Build history of the part. All positions in model axes, mm. Face numbers are marked on the shaded views. A direction names the side the tool comes from. Round coordinates to 2 decimals unless told otherwise and drop trailing zeros. Write each loop counter-clockwise with the first axis right and the second up, starting at its lowest first coordinate (ties: lowest second). Pieces come first, ordered by that corner, then holes. Notation, with made-up numbers: (-31, 54.5) -> (-17, 54.5) arc R26 ccw to (-17, 84.5) -> close; hole circle Ø1 at (26.25, -33). An arc over 180 degrees is marked (long way). Answer in a Markdown table with one row per item. Add a question column.
from build123d import *

# Parameters (mm, degrees)
SKETCH1_R           = 3
SKETCH1_R_2         = 1.6
BOSS_EXTRUDE1_DEPTH = 3


with BuildPart() as part:
    # Sketch1 → Boss-Extrude1 (new body)
    with BuildSketch(Plane(origin=(0, 0, 0), x_dir=(1, 0, 0), z_dir=(0, 1, 0))):
        with BuildLine():
            Line((-4.898979486, 26), (-9.797958971, 2))
            ThreePointArc((-9.797958971, 2), (0, -10), (9.797958971, 2))
            Line((9.797958971, 2), (4.898979486, 26))
            ThreePointArc((4.898979486, 26), (0, 30), (-4.898979486, 26))
        make_face()
        with Locations(Location((0, 0, 0), (0, 0, 270))):
            Circle(SKETCH1_R, mode=Mode.SUBTRACT)
        with Locations(Location((0, 7, 0), (0, 0, 270))):
            Circle(SKETCH1_R_2, mode=Mode.SUBTRACT)
        with Locations(Location((7, 0, 0), (0, 0, 270))):
            Circle(SKETCH1_R_2, mode=Mode.SUBTRACT)
        with Locations(Location((0, -7, 0), (0, 0, 270))):
            Circle(SKETCH1_R_2, mode=Mode.SUBTRACT)
        with Locations(Location((-7, 0, 0), (0, 0, 270))):
            Circle(SKETCH1_R_2, mode=Mode.SUBTRACT)
        with BuildLine():
            Line((1.6, 25), (1.6, 20))
            ThreePointArc((1.6, 20), (0, 18.4), (-1.6, 20))
            Line((-1.6, 20), (-1.6, 25))
            ThreePointArc((-1.6, 25), (0, 26.6), (1.6, 25))
        make_face(mode=Mode.SUBTRACT)
    extrude(amount=BOSS_EXTRUDE1_DEPTH)


solid = part.part
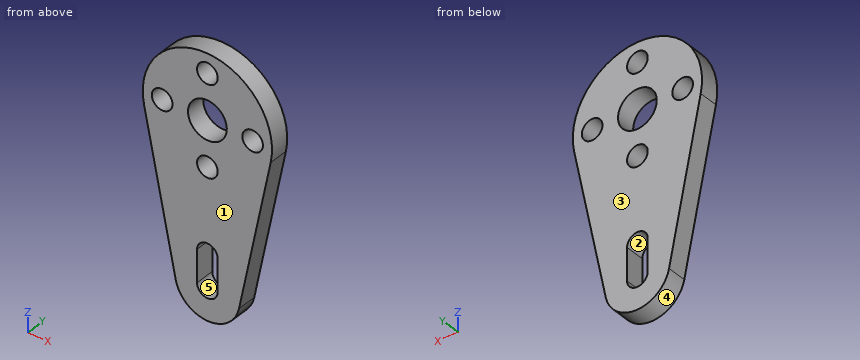
(1) Drop flat-ended pins along their axis: P1, Ø1, axis at y = 1.5, z = -25.5, coming from the +X side; P2, Ø1.5, axis at x = 5.5, y = 2, coming from the +Z side; P3, Ø1.5, axis at y = 1, z = -22, coming from the +X side. Give the stop position or say it passes through.
(2) Saw through at C-C (z = -6). List the corners of the cut face in (x, y).
(3) Probe line 1 along X through (y, z) = (1.7, 0); line 2 along Z through (x, y) = (0.25, 1.7); line 3 along Z through (x, y) = (1.75, 1.35). List the from-to ranges inside material, lowest first.
(4) Saw through at A-A (y = 1.15). List the corners of the cut face in (x, z).
(5) Saw through at B-B (x = 0). List the corners of the cut face in (y, z), plus the area to 3 significant figures.
(6) Saw through at D-D (x = -7). List the corners of the cut face in (y, z).
(7) Which spindle directions (+Z, -Z, +X, -X, +Y, -Y) get a long thin tool onto all of the face, cutting with end or side? Do the marked faces 1 and 2. Say none if no direction does.
(8) Mould opens along Z. For the marked faces 3, 4 and 5 say: pulls with the +Z half, pulls with the -Z half, needs draft (parallel to the pull), parting line crosses it, or undercut.
Answer sheet:
| question | item | result |
|---|---|---|
| 1 | P1 | stops at x = 5.1 |
| 1 | P2 | stops at z = 8.8 |
| 1 | P3 | stops at x = 5.87 |
| 2 | outline | (-8.98, 0) -> (-1.25, 0) -> (-1.25, 3) -> (-8.98, 3) -> close; (1.25, 0) -> (8.98, 0) -> (8.98, 3) -> (1.25, 3) -> close |
| 3 | line 1 | x = -10 to -8.6, -5.4 to -3, 3 to 5.4, 8.6 to 10 |
| 3 | line 2 | z = -29.99 to -26.58, -18.42 to -8.58, -5.42 to -2.99, 2.99 to 5.42, 8.58 to 10 |
| 3 | line 3 | z = -29.68 to -2.44, 2.44 to 9.85 |
| 4 | outline | (-9.8, -2) -> (-4.9, -26) arc R5 ccw to (4.9, -26) -> (9.8, -2) arc R10 ccw (long way) to start; hole circle Ø3.2 at (-7, 0); hole circle Ø6 at (0, 0); hole (-1.6, -25) arc R1.6 ccw to (1.6, -25) -> (1.6, -20) arc R1.6 ccw to (-1.6, -20) -> close; hole circle Ø3.2 at (0, -7); hole circle Ø3.2 at (0, 7); hole circle Ø3.2 at (7, 0) |
| 5 | outline | (0, -30) -> (3, -30) -> (3, -26.6) -> (0, -26.6) -> close; (0, -18.4) -> (3, -18.4) -> (3, -8.6) -> (0, -8.6) -> close; (0, -5.4) -> (3, -5.4) -> (3, -3) -> (0, -3) -> close; (0, 3) -> (3, 3) -> (3, 5.4) -> (0, 5.4) -> close; (0, 8.6) -> (3, 8.6) -> (3, 10) -> (0, 10) -> close |
| 5 | area | 58.2 mm² |
| 6 | outline | (0, -15.71) -> (3, -15.71) -> (3, -1.6) -> (0, -1.6) -> close; (0, 1.6) -> (3, 1.6) -> (3, 7.14) -> (0, 7.14) -> close |
| 7 | face 1 | +Z, -Z, +X, -X, -Y |
| 7 | face 2 | +Y, -Y |
| 8 | face 3 | needs draft |
| 8 | face 4 | pulls with the -Z half |
| 8 | face 5 | undercut |
